from build123d import *

# Parameters (mm, degrees)
ESQUISSE1_W             = 50
ESQUISSE1_H             = 94
ESQUISSE1_R             = 11
ESQUISSE1_R_2           = 2
BOSS_EXTRU_1_DEPTH      = 8
CHANFREIN1_SIZE         = 2.5
ESQUISSE2_R             = 2
ENL_V_MAT_EXTRU_1_DEPTH = 10
ESQUISSE3_R             = 8
ENL_V_MAT_EXTRU_2_DEPTH = 5
ESQUISSE4_R             = 3
ENL_V_MAT_EXTRU_3_DEPTH = 79.852413099
ESQUISSE5_W             = 50
ESQUISSE5_H             = 8
ENL_V_MAT_EXTRU_4_DEPTH = 2


with BuildPart() as part:
    # Esquisse1 → Boss.-Extru.1 (new body)
    with BuildSketch(Plane(origin=(0, 0, 0), x_dir=(1, 0, 0), z_dir=(0, 1, 0))):
        with Locations((-6.491408935, -25.117918819)):
            Rectangle(ESQUISSE1_W, ESQUISSE1_H)
        with Locations(Location((-6.491408935, 6.882081181, 0), (0, 0, 270))):
            Circle(ESQUISSE1_R, mode=Mode.SUBTRACT)
        with Locations(Location((-26.491408935, -19.117918819, 0), (0, 0, 270))):
            Circle(ESQUISSE1_R_2, mode=Mode.SUBTRACT)
        with Locations(Location((13.508591065, -19.117918819, 0), (0, 0, 270))):
            Circle(ESQUISSE1_R_2, mode=Mode.SUBTRACT)
    extrude(amount=BOSS_EXTRU_1_DEPTH)

    # Chanfrein1
    chanfrein1_edges = [part.edges().sort_by_distance(p)[0] for p in [
        (-26.491408935, 8, 17.117918819),
        (13.508591065, 8, 17.117918819),
    ]]
    chamfer(chanfrein1_edges, length=CHANFREIN1_SIZE)

    # Esquisse2 → Enlèv. mat.-Extru.1 (cut)
    with BuildSketch(Plane.XY.offset(72.117918819)):
        with Locations((-21.491408935, 4)):
            Circle(ESQUISSE2_R)
        with Locations((8.508591065, 4)):
            Circle(ESQUISSE2_R)
    extrude(amount=-ENL_V_MAT_EXTRU_1_DEPTH, mode=Mode.SUBTRACT)

    # Esquisse3 → Enlèv. mat.-Extru.2 (cut)
    with BuildSketch(Plane.XZ):
        with Locations(Location((-6.491408935, 56.117918819, 0), (0, 0, 270))):
            Circle(ESQUISSE3_R)
    extrude(amount=-ENL_V_MAT_EXTRU_2_DEPTH, mode=Mode.SUBTRACT)

    # Esquisse4 → Enlèv. mat.-Extru.3 (cut, through all)
    with BuildSketch(Plane.XZ.offset(-5)):
        with Locations(Location((-6.491408935, 56.117918819, 0), (0, 0, 270))):
            Circle(ESQUISSE4_R)
    extrude(amount=-ENL_V_MAT_EXTRU_3_DEPTH, mode=Mode.SUBTRACT)

    # Esquisse5 → Enlèv. mat.-Extru.4 (cut)
    with BuildSketch(Plane.XZ):
        with Locations((-6.491408935, 19.117918819)):
            Rectangle(ESQUISSE5_W, ESQUISSE5_H)
    extrude(amount=-ENL_V_MAT_EXTRU_4_DEPTH, mode=Mode.SUBTRACT)


solid = part.part
Could you check a few things on this model? Use its own coordinates, in mm. A direction names the side the tool comes from. Give positions to 0.01 mm unless a question says otherwise; leave off trailing zeros. Order: outer loops, then holes, each group sorted by start corner. A loop starts at its lowest first (then second) coordinate and runs counter-clockwise, first axis right, second up.
1. Will these pins go through, and if not, where does the flat tip stop? P1, Ø3, axis at x = -15, z = 27, coming from the -Y side; P2, Ø6.5, axis at x = 13.51, z = 19.12, coming from the -Y side; P3, Ø5, axis at x = -6.49, z = 56.12, coming from the -Y side; P4, Ø3, axis at x = -21.49, y = 4, coming from the +Z side.
2. Suppose I cut it at B-B (z = 58). List the corners of the cut face in (x, y) for me.
3. For faces 1 (the flat face through (18.509, 4, 26)), 2 (the flat face through (-6, 5, 53)), 3 (the flat face through (8, 4, 62.118)), 4 (the flat face through (-7, 1, 15.118)), which set-ups out of +Z, -Z, +X, -X, +Y, -Y let a thin tool reach every point of the face, with its end or its side?
4. Suppose I cut it at A-A (x = -12.5). List the corners of the cut face in (y, z) for me.
5. Suppose I cut it at C-C (y = 3). List the corners of the cut face in (x, z) for me.
6. We'd pull the mould along Y, two halves only. Please class faces 5 (the conical face through (-28.6, 5.66, 18.65)), 6 (the cylindrical face through (-6.36, 6.479, 59.115)), 7 (the cylindrical face through (-21.925, 2.048, 67.188)), 8 (the flat face through (-22, 4, 62.118)): pulls with the +Y half, pulls with the -Y half, needs draft (parallel to the pull), parting line crosses it, or undercut.
7. Suppose I cut it at D-D (x = -20.5). List the corners of the cut face in (y, z) for me.
8. I need wall thicknesses on L1, parallel to Z at x = -9, y = 7.5; L2, parallel to Z at x = 6, y = 1.25; L3, parallel to Z at x = -8.5, y = 1. Which ranges of each line are inside material? Lowest first, please.
Solved:
1. P1: stops at y = 0
1. P2: stops at y = 2
1. P3: passes through
1. P4: stops at z = 62.12
2. outline: (-31.49, 0) - (-14.27, 0) - (-14.27, 5) - (-8.83, 5) - (-8.83, 8) - (-31.49, 8) - close; (-4.16, 5) - (1.28, 5) - (1.28, 0) - (18.51, 0) - (18.51, 8) - (-4.16, 8) - close
3. face 1: +Z, -Z, +X, +Y, -Y
3. face 2: -Y
3. face 3: +Z
3. face 4: +X, -X, -Y
4. outline: (0, -21.88) - (8, -21.88) - (8, -16.1) - (0, -16.1) - close; (0, 2.33) - (8, 2.33) - (8, 72.12) - (0, 72.12) - (0, 61.4) - (5, 61.4) - (5, 50.84) - (0, 50.84) - (0, 23.12) - (2, 23.12) - (2, 15.12) - (0, 15.12) - close
5. outline: (-31.49, -21.88) - (18.51, -21.88) - (18.51, 72.12) - (10.24, 72.12) - (10.24, 62.12) - (6.78, 62.12) - (6.78, 72.12) - (-19.76, 72.12) - (-19.76, 62.12) - (-23.22, 62.12) - (-23.22, 72.12) - (-31.49, 72.12) - close; hole circle Ø4 at (-26.49, 19.12); hole circle Ø22 at (-6.49, -6.88); hole circle Ø16 at (-6.49, 56.12); hole circle Ø4 at (13.51, 19.12)
6. face 5: pulls with the +Y half
6. face 6: needs draft
6. face 7: undercut
6. face 8: undercut
7. outline: (0, -21.88) - (8, -21.88) - (8, 72.12) - (5.74, 72.12) - (5.74, 62.12) - (2.26, 62.12) - (2.26, 72.12) - (0, 72.12) - (0, 23.12) - (2, 23.12) - (2, 15.12) - (0, 15.12) - close
8. L1: z = -21.88 to -17.59, 3.83 to 54.47, 57.76 to 72.12
8. L2: z = -21.88 to 15.12, 23.12 to 72.12
8. L3: z = -21.88 to -17.7, 3.93 to 15.12, 23.12 to 48.37, 63.86 to 72.12
